from build123d import *

# Parameters (mm, degrees)
SZKIC1_R                    = 6
DODANIE_WYCI_GNI_CIE1_DEPTH = 60
DODANIE_WYCI_GNI_CIE2_DEPTH = 5.5
SFAZOWANIE1_SIZE            = 1
SZKIC6_R                    = 9.75
SZKIC6_R_2                  = 6.5
DODANIE_WYCI_GNI_CIE3_DEPTH = 2.5


with BuildPart() as part:
    # Szkic1 → Dodanie-wyciągnięcie1 (new body)
    with BuildSketch(Plane(origin=(0, 0, 0), x_dir=(1, 0, 0), z_dir=(0, 1, 0))):
        with Locations(Location((0, 0, 0), (0, 0, 270))):
            Circle(SZKIC1_R)
    extrude(amount=-DODANIE_WYCI_GNI_CIE1_DEPTH)

    # Szkic2 → Dodanie-wyciągnięcie2 (add)
    with BuildSketch(Plane(origin=(0, 0, 0), x_dir=(1, 0, 0), z_dir=(0, 1, 0))):
        Polygon((10.969655115, 0), (5.484827557, 9.5), (-5.484827557, 9.5), (-10.969655115, 0), (-5.484827557, -9.5), (5.484827557, -9.5), align=None)
    extrude(amount=DODANIE_WYCI_GNI_CIE2_DEPTH)

    # Szkic4 → Wycięcie-obrót1 (revolve, cut)
    with BuildSketch(Plane.XY):
        Polygon((10.969655115, 4.030344885), (9.5, 5.5), (10.969655115, 5.5), align=None)
    revolve(axis=Axis((0, 5.5, 0), (0, -1, 0)), mode=Mode.SUBTRACT)

    # Sfazowanie1
    sfazowanie1_edges = [part.edges().sort_by_distance(p)[0] for p in [
        (0, -60, -6),
    ]]
    chamfer(sfazowanie1_edges, length=SFAZOWANIE1_SIZE)

    # Szkic6 → Dodanie-wyciągnięcie3 (add)
    with BuildSketch(Plane.XZ):
        with Locations(Location((0, 0, 0), (0, 0, 76.997175533))):
            Circle(SZKIC6_R)
        with Locations(Location((0, 0, 0), (0, 0, 270))):
            Circle(SZKIC6_R_2, mode=Mode.SUBTRACT)
    extrude(amount=DODANIE_WYCI_GNI_CIE3_DEPTH)


solid = part.part
The listing builds one solid part. Answer for the finished solid, in the listing's coordinates (mm). A direction names the side the tool comes from. Coordinates: 2 decimals unless noted, no trailing zeros. Order: outer loops, then holes, each group sorted by start corner. A loop starts at its lowest first (then second) coordinate and runs counter-clockwise, first axis right, second up. Notation, with made-up numbers: (12, 31) -> (31, 31) arc R24 ccw to (31, 44) -> close; hole circle Ø7 at (-36.5, -24). An arc over 180 degrees is marked (long way). Answer in a Markdown table with one row per item. Add a question column.
Item 1: Determine the mould class of faces 1 (the face through (-3.955, -1.232, 5.158)), 2 (the face through (0, -60, 0)), 3 (the face through (-10, 5, 0)), 4 (the face through (-4.904, 5.15, 8.543)) for opening direction Z: +Z half, -Z half, draft (parallel to the pull), parting line (faces both ways), or undercut.
Item 2: Which of the six approach directions +Z, -Z, +X, -X, +Y, -Y give full straight-line access (tool end or side, diameter ignored) to faces 5 (the face through (5, 0, -9)), 6 (the face through (5, 0, 9)), 7 (the face through (-5, 0, 9)), 8 (the face through (-8.266, 2.711, 4.684))?
Item 3: Find the intervals of material crossed by L1, parallel to X at y = -2, z = 0; L2, parallel to Y at x = -4.5, z = 5.5; L3, parallel to X at y = 1, z = 7.5, in increasing order. Write a range as from..to.
Item 4: Each of these flat-tipped pins is pushed along its axis until it touches: P1, Ø1.5, axis at x = 5.5, z = -3.5, coming from the -Y side; P2, Ø0.9, axis at x = -5, z = -8.5, coming from the -Y side; P3, Ø4.5, axis at x = 2, y = 1.5, coming from the -Z side. Where does it stop, or does it pass through?
Item 5: Find section A-A (y = -11). Write down the section's boundary in (x, z).
Result set:
| question | item | result |
|---|---|---|
| 1 | face 1 | undercut |
| 1 | face 2 | draft |
| 1 | face 3 | parting line |
| 1 | face 4 | +Z half |
| 2 | face 5 | -Z, +X, -Y |
| 2 | face 6 | +Z, +X, -Y |
| 2 | face 7 | +Z, -X, -Y |
| 2 | face 8 | +Z, -X, +Y |
| 3 | L1 | x = -9.75..-6.5, -6..6, 6.5..9.75 |
| 3 | L2 | y = -2.5..5.5 |
| 3 | L3 | x = -6.64..6.64 |
| 4 | P1 | stops at y = -59.23 |
| 4 | P2 | stops at y = -2.5 |
| 4 | P3 | stops at z = -9.74 |
| 5 | outline | circle Ø12 at (0, 0) |
